Model file for the job. Use its own axes, mm. Face numbers are marked on the shaded views. Give positions to 0.01 mm unless a question says otherwise; leave off trailing zeros. Order: outer loops, then holes, each group sorted by start corner. A loop starts at its lowest first (then second) coordinate and runs counter-clockwise, first axis right, second up. Notation, with made-up numbers: (-32, -12) - (-6, -12) arc R28 cw to (-6, 11) - close; hole circle Ø3 at (57, 58). An arc over 180 degrees is marked (long way). Use CSV: the item, a comma, the result in double quotes. Start each with the question number.
(1) Probe L1, parallel to Y at x = -24, z = 76; L2, parallel to Z at x = -55.5, y = 24; L3, parallel to X at y = 22, z = 80.5. List the from-to ranges inside material, lowest first.
(2) Band-saw the part on B-B, the plane y = 65.5. Give the cut face in (x, z).
(3) Band-saw the part on C-C, the plane z = 112. Give the cut face in (x, y).
(4) Pull direction Y, two halves, no side cores. Call the marked faces 1 and 2: +Y half, -Y half, draft (parallel to the pull), parting line (faces both ways), or undercut.
(5) Drop flat-ended pins along their axis: pin 1 Ø4 at (x, z) = (-18, 77) entering from -Y; pin 2 Ø11.5 at (y, z) = (-43, 57) entering from -X; pin 3 Ø12 at (y, z) = (-25.5, 60.5) entering from +X; pin 4 Ø10 at (x, z) = (-20.5, 84.5) entering from +Y. Give the stop position or say it passes through.
(6) Band-saw the part on D-D, the plane y = 25. Give the cut face in (x, z).
(7) Band-saw the part on A-A, the plane x = -75. Give the cut face in (y, z), then the cut area to 3 significant figures.
from build123d import *

# Parameters (mm, degrees)
F1_DEPTH  = 127
F2_W      = 88.9
F2_H      = 114.3
F3_DEPTH  = 152.6319465885
F5_DEPTH  = 12.7
F9_DEPTH  = 12.7
F10_DEPTH = 12.7


with BuildPart() as f1:
    # F0 (on Top) → F1 (new body)
    with BuildSketch(Plane.XY):
        Polygon((0, -76.2), (0, 0), (0, 76.2), (-101.6, 76.4309465885), (-101.6, -76.2), align=None)
    extrude(amount=F1_DEPTH)

    # F2 (on face) → F3 (cut, through all)
    with BuildSketch(Plane.XZ.offset(76.2)):
        with Locations((-57.15, 69.85)):
            Rectangle(F2_W, F2_H)
    extrude(amount=-F3_DEPTH, mode=Mode.SUBTRACT)

    # F4 (on face) → F5 (join)
    with BuildSketch(Plane.XZ.offset(76.2)):
        Polygon((-12.7, 127), (-101.6, 12.7), (-93.1919366121, 12.7), (-12.7, 116.189632787), align=None)
    extrude(amount=-F5_DEPTH)

    # F6: F1 across plane


with BuildPart() as f1_1:
    add(f1.part)
    add(f1.part.mirror(Plane.XZ))

    # F8 (on face) → F9 (join)
    with BuildSketch(Plane(origin=(-12.7, 0, 0), x_dir=(0, -1, 0), z_dir=(-1, 0, 0))):
        Polygon((27.0305331796, 108.3241701126), (18.2572510093, 105.0341874361), (21.9403224368, 79.9026338657), (14.9672674015, 84.8556309938), (21.9403224368, 53.9298020303), (15.4059324414, 57.6584488153), (23.1189505014, 23.4508488309), (23.1189505014, 48.2271686196), (28.1271934509, 41.8665371835), (25.9338729084, 73.0116963387), (30.9785138816, 65.1157423854), (30.3082256371, 72.4516701299), (27.5382939124, 102.7670145489), align=None)
        with BuildLine():
            ThreePointArc((30.9785138816, 65.1157423854), (53.7975454705, 88.9853099615), (27.0305331796, 108.3241701126))
            Line((27.0305331796, 108.3241701126), (27.5382939124, 102.7670145489))
            ThreePointArc((27.5382939124, 102.7670145489), (46.803503681, 89.2430712576), (30.3082256371, 72.4516701299))
            Line((30.3082256371, 72.4516701299), (30.9785138816, 65.1157423854))
        make_face()
    extrude(amount=F9_DEPTH)

    # F7 (on face) → F10 (join)
    with BuildSketch(Plane(origin=(-12.7, 0, 0), x_dir=(0, -1, 0), z_dir=(-1, 0, 0))):
        with BuildLine():
            Line((-41.1189049482, 55.9498922817), (-41.1189049482, 60.0139613671))
            ThreePointArc((-41.1189049482, 60.0139613671), (-46.1180179766, 60.8526580466), (-50.9355384856, 62.4293759465))
            Line((-50.9355384856, 62.4293759465), (-48.3765341341, 66.3066580892))
            Line((-48.3765341341, 66.3066580892), (-53.4945428371, 62.8946498036))
            ThreePointArc((-53.4945428371, 62.8946498036), (-47.8245334602, 58.4995284296), (-41.1189049482, 55.9498922817))
        make_face()
        with BuildLine():
            Line((-33.9530482888, 95.3087136149), (-41.1189049482, 95.3087136149))
            Line((-41.1189049482, 95.3087136149), (-41.1189049482, 60.0139613671))
            ThreePointArc((-41.1189049482, 60.0139613671), (-37.5331179531, 59.8773300828), (-33.9530482888, 60.1215383586))
            Line((-33.9530482888, 60.1215383586), (-33.9530482888, 60.6629624963))
            Line((-33.9530482888, 60.6629624963), (-33.9530482888, 95.3087136149))
        make_face()
        with BuildLine():
            ThreePointArc((-33.9530482888, 55.4682547852), (-37.5538538559, 55.4430939924), (-41.1189049482, 55.9498922817))
            Line((-41.1189049482, 55.9498922817), (-41.1189049482, 25.4587136149))
            Line((-41.1189049482, 25.4587136149), (-33.9530482888, 25.4587136149))
            Line((-33.9530482888, 25.4587136149), (-33.9530482888, 55.4682547852))
        make_face()
        with BuildLine():
            ThreePointArc((-33.9530482888, 60.1215383586), (-37.5331179531, 59.8773300828), (-41.1189049482, 60.0139613671))
            Line((-41.1189049482, 60.0139613671), (-41.1189049482, 55.9498922817))
            ThreePointArc((-41.1189049482, 55.9498922817), (-37.5538538559, 55.4430939924), (-33.9530482888, 55.4682547852))
            Line((-33.9530482888, 55.4682547852), (-33.9530482888, 60.1215383586))
        make_face()
        with BuildLine():
            ThreePointArc((-20.7989049482, 64.6006539464), (-27.1433610579, 61.6779571784), (-33.9530482888, 60.1215383586))
            Line((-33.9530482888, 60.1215383586), (-33.9530482888, 55.4682547852))
            ThreePointArc((-33.9530482888, 55.4682547852), (-26.9900318901, 57.0883116374), (-20.7989049482, 60.6629624963))
            Line((-20.7989049482, 60.6629624963), (-20.7989049482, 64.6006539464))
        make_face()
        Polygon((-20.7989049482, 98.4088753533), (-20.7989049482, 64.6006539464), (-20.7989049482, 60.6629624963), (-20.7989049482, 22.2088753533), (-13.1789049482, 22.2088753533), (-13.1789049482, 62.8946498036), (-13.1789049482, 70.8043053746), (-13.1789049482, 98.4088753533), align=None)
        with BuildLine():
            ThreePointArc((-2.1593503188, 70.8043053746), (-7.6691276335, 71.4665793512), (-13.1789049482, 70.8043053746))
            Line((-13.1789049482, 70.8043053746), (-13.1789049482, 62.8946498036))
            ThreePointArc((-13.1789049482, 62.8946498036), (-9.105292791, 65.0897069065), (-4.640808329, 66.3066580892))
            Line((-4.640808329, 66.3066580892), (-2.1593503188, 70.8043053746))
        make_face()
    extrude(amount=F10_DEPTH)


solid = f1_1.part
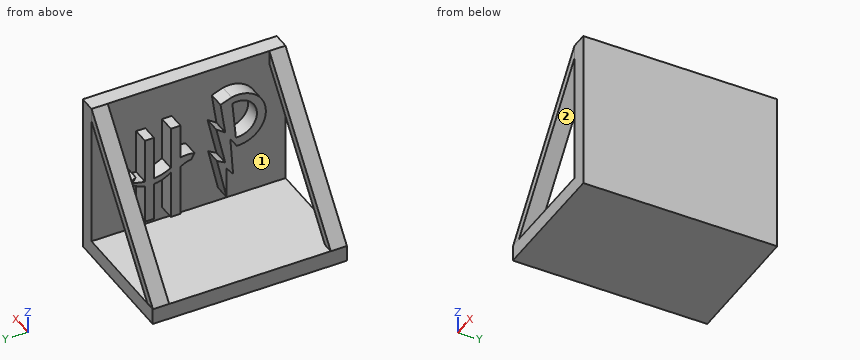
Answer block:
1,L1,"y = -50.93 to -41.33, -29.98 to -16.96, 13.18 to 20.8, 33.95 to 41.12"
1,L2,"z = 0 to 12.7"
1,L3,"x = -12.7 to 0"
2,outline,"(-101.6, 0) - (0, 0) - (0, 127) - (-12.7, 127) - (-101.6, 12.7) - close; hole (-93.19, 12.7) - (-12.7, 12.7) - (-12.7, 116.19) - close"
3,outline,"(-24.37, -76.2) - (-15.96, -76.2) - (-15.96, -63.5) - (-24.37, -63.5) - close; (-24.37, 63.5) - (-15.96, 63.5) - (-15.96, 76.2) - (-24.37, 76.2) - close; (-12.7, -76.23) - (0, -76.2) - (0, 76.2) - (-12.7, 76.23) - close"
4,face 1,"undercut"
4,face 2,"draft"
5,pin 1,"stops at y = -52.38"
5,pin 2,"stops at x = -12.7"
5,pin 3,"stops at x = 0"
5,pin 4,"stops at y = 41.12"
6,outline,"(-101.6, 0) - (0, 0) - (0, 127) - (-12.7, 127) - (-12.7, 62.49) - (-25.4, 62.49) - (-25.4, 57.98) - (-12.7, 57.98) - (-12.7, 12.7) - (-101.6, 12.7) - close"
7,outline,"(-76.37, 0) - (76.37, 0) - (76.37, 12.7) - (-76.37, 12.7) - close; (-76.2, 36.09) - (-63.5, 36.09) - (-63.5, 46.9) - (-76.2, 46.9) - close; (63.5, 36.09) - (76.2, 36.09) - (76.2, 46.9) - (63.5, 46.9) - close"
7,area,"2,210 mm2"
